```python
from build123d import *

# Parameters (mm, degrees)
SKETCH1_W               = 14.59562339
SKETCH1_H               = 8.02
SKETCH1_R               = 1.625
BOSS_EXTRUDE1_DEPTH     = 3.25
SKETCH2_W               = 14.59562339
SKETCH2_H               = 5.77
CUT_EXTRUDE1_DEPTH      = 2.4
CUT_EXTRUDE2_DEPTH      = 4.25
CUT_EXTRUDE2_DEPTH_BACK = 4.25
FILLET1_R               = 0.5


with BuildPart() as part:
    # Sketch1 → Boss-Extrude1 (new body, symmetric)
    with BuildSketch(Plane(origin=(0, 0, 0), x_dir=(0, 0, -1), z_dir=(1, 0, 0))):
        Rectangle(SKETCH1_W, SKETCH1_H)
        with Locations((-5.277811695, 1.5)):
            Circle(SKETCH1_R, mode=Mode.SUBTRACT)
        with Locations((2.222188305, 1.5)):
            Circle(SKETCH1_R, mode=Mode.SUBTRACT)
    extrude(amount=BOSS_EXTRUDE1_DEPTH, both=True)

    # Sketch2 → Cut-Extrude1 (cut, symmetric)
    with BuildSketch(Plane(origin=(0, 0, 0), x_dir=(0, 0, -1), z_dir=(1, 0, 0))):
        with Locations((0, 1.125)):
            Rectangle(SKETCH2_W, SKETCH2_H)
    extrude(amount=CUT_EXTRUDE1_DEPTH, both=True, mode=Mode.SUBTRACT)

    # Sketch4 → Cut-Extrude2 (cut, two sides)
    with BuildSketch(Plane(origin=(0, 0, 0), x_dir=(0, 0, -1), z_dir=(1, 0, 0))) as cut_extrude2_sk:
        with BuildLine():
            Line((4.047811695, 4.01), (7.297811695, 4.01))
            Line((7.297811695, 4.01), (7.297811695, 0.76))
            ThreePointArc((7.297811695, 0.76), (4.999714656, 1.711902961), (4.047811695, 4.01))
        make_face()
    extrude(amount=CUT_EXTRUDE2_DEPTH, mode=Mode.SUBTRACT)
    extrude(cut_extrude2_sk.sketch, amount=-CUT_EXTRUDE2_DEPTH_BACK, mode=Mode.SUBTRACT)

    # Fillet1
    fillet1_edges = [part.edges().sort_by_distance(p)[0] for p in [
        (2.825, 0.76, -7.297811695),
        (2.825, 4.01, -4.047811695),
        (-2.825, 0.76, -7.297811695),
        (-2.825, 4.01, -4.047811695),
    ]]
    fillet(fillet1_edges, radius=FILLET1_R)


solid = part.part
```
Read the model definition and answer for the solid it produces. Units are mm, in the model's axes. A direction names the side the tool comes from. Give positions to 0.01 mm unless a question says otherwise; leave off trailing zeros. Loops run counter-clockwise (first coordinate to the right, second up) from the corner with the lowest first, then second, coordinate; pieces in that order, holes last.
Item 1: For faces 5 (the flat face through (2.4, 1, 0)), 6 (the cylindrical face through (2.819, 0.511, 6.567)), determine the directions among +Z, -Z, +X, -X, +Y, -Y from which every point of the face is accessible in a straight line to the end or side of a thin tool.
Item 2: The part is cut by section C-C (z = 6.25). Write down the section's boundary in (x, y), and give its area (3 significant figures).
Item 3: The part is cut by section A-A (x = 3). Write down the section's boundary in (y, z) (3 decimals).
Item 4: Find the intervals of material crossed by line 1 along X through (y, z) = (3.75, 0.25); line 2 along Z through (x, y) = (2.9, 1.5); line 3 along Y through (x, z) = (1.75, 6), in increasing order.
Item 5: The part is cut by section B-B (y = -0.5). Write down the section's boundary in (x, z), and give its area (3 significant figures).
Item 6: The mould has two halves that part along Y. Classify faces 1 (the flat face through (-2.4, 1, 0)), 2 (the cylindrical face through (2.82, 1.69, -5.02)), 3 (the flat face through (0, -4.01, 0)), 4 (the cylindrical face through (-2.831, 0.511, 6.567)): released by +Y, released by -Y, zero draft, split by the parting line, or undercut.
Item 7: This flat-tipped pin is pushed along its axis until it touches: pin 1 Ø3.5 at (y, z) = (1.5, 5.28) entering from -X. Where does it stop, or does it pass through?
Item 8: The part is cut by section D-D (y = 2.25). Write down the section's boundary in (x, z), and give its area (3 significant figures).
Taken from the geometry:
1. face 5: +Z, -Z, +Y
1. face 6: +X, -X
2. outline: (-3.25, -4.01) - (3.25, -4.01) - (3.25, 0.2) - (2.4, 0.2) - (2.4, -1.76) - (-2.4, -1.76) - (-2.4, 0.2) - (-3.25, 0.2) - close; (-3.25, 2.8) - (-2.4, 2.8) - (-2.4, 4.01) - (-3.25, 4.01) - close; (2.4, 2.8) - (3.25, 2.8) - (3.25, 4.01) - (2.4, 4.01) - close
2. area: 20.0 mm2
3. outline: (-4.01, -7.298) - (0.293, -7.298) arc R0.5 ccw to (0.789, -6.864) arc R3.25 cw to (3.577, -4.077) arc R0.5 ccw to (4.01, -3.581) - (4.01, 7.298) - (-4.01, 7.298) - close; hole circle Ø3.25 at (1.5, -2.222); hole circle Ø3.25 at (1.5, 5.278)
4. line 1: x = -3.25 to -2.4, 2.4 to 3.25
4. line 2: z = -5.23 to -3.85, -0.6 to 3.65, 6.9 to 7.3
4. line 3: y = -4.01 to -1.76
5. outline: (-3.25, -7.3) - (-2.4, -7.3) - (-2.4, 7.3) - (-3.25, 7.3) - close; (2.4, -7.3) - (3.25, -7.3) - (3.25, 7.3) - (2.4, 7.3) - close
5. area: 24.8 mm2
6. face 1: zero draft
6. face 2: released by +Y
6. face 3: released by -Y
6. face 4: undercut
7. pin 1: stops at x = -3.25
8. outline: (-3.25, -4.57) - (-2.4, -4.57) - (-2.4, -3.66) - (-3.25, -3.66) - close; (-3.25, -0.78) - (-2.4, -0.78) - (-2.4, 3.84) - (-3.25, 3.84) - close; (-3.25, 6.72) - (-2.4, 6.72) - (-2.4, 7.3) - (-3.25, 7.3) - close; (2.4, -4.57) - (3.25, -4.57) - (3.25, -3.66) - (2.4, -3.66) - close; (2.4, -0.78) - (3.25, -0.78) - (3.25, 3.84) - (2.4, 3.84) - close; (2.4, 6.72) - (3.25, 6.72) - (3.25, 7.3) - (2.4, 7.3) - close
8. area: 10.4 mm2
